from build123d import *

# Parameters (mm, degrees)
F1_DEPTH = 50.8
F3_DEPTH = 76.2
F4_R     = 38.1
F5_DEPTH = 12.7
F6_R     = 9.525
F7_DEPTH = 25.401


with BuildPart() as f1:
    # F0 (on Front) → F1 (new body, symmetric)
    with BuildSketch(Plane.XZ):
        with BuildLine():
            ThreePointArc((-92.075, -61.1803239805), (-60.325, -61.1803239805), (-44.45, -88.6766305507))
            Line((-44.45, -88.6766305507), (44.45, -88.6766305507))
            ThreePointArc((44.45, -88.6766305507), (60.325, -61.1803239805), (92.075, -61.1803239805))
            Line((92.075, -61.1803239805), (159.3117036526, 55.2770628791))
            ThreePointArc((159.3117036526, 55.2770628791), (147.6903970824, 66.8983694493), (143.4367036526, 82.7733694493))
            Line((143.4367036526, 82.7733694493), (-143.4367036526, 82.7733694493))
            ThreePointArc((-143.4367036526, 82.7733694493), (-147.6903970824, 66.8983694493), (-159.3117036526, 55.2770628791))
            Line((-159.3117036526, 55.2770628791), (-92.075, -61.1803239805))
        make_face()
        with BuildLine():
            Line((-168.8367036526, 71.7748468212), (-159.3117036526, 55.2770628791))
            ThreePointArc((-159.3117036526, 55.2770628791), (-147.6903970824, 66.8983694493), (-143.4367036526, 82.7733694493))
            Line((-143.4367036526, 82.7733694493), (-162.4867036526, 82.7733694493))
            ThreePointArc((-162.4867036526, 82.7733694493), (-164.1881810245, 76.4233694493), (-168.8367036526, 71.7748468212))
        make_face()
        with BuildLine():
            ThreePointArc((-143.4367036526, 82.7733694493), (-202.6830102227, 98.6483694493), (-159.3117036526, 55.2770628791))
            Line((-159.3117036526, 55.2770628791), (-168.8367036526, 71.7748468212))
            ThreePointArc((-168.8367036526, 71.7748468212), (-186.1852262806, 89.1233694493), (-162.4867036526, 82.7733694493))
            Line((-162.4867036526, 82.7733694493), (-143.4367036526, 82.7733694493))
        make_face()
        with BuildLine():
            Line((168.8367036526, 71.7748468212), (159.3117036526, 55.2770628791))
            ThreePointArc((159.3117036526, 55.2770628791), (191.0617036526, 55.2770628791), (206.9367036526, 82.7733694493))
            ThreePointArc((206.9367036526, 82.7733694493), (175.1867036526, 114.5233694493), (143.4367036526, 82.7733694493))
            Line((143.4367036526, 82.7733694493), (162.4867036526, 82.7733694493))
            ThreePointArc((162.4867036526, 82.7733694493), (175.1867036526, 95.4733694493), (187.8867036526, 82.7733694493))
            ThreePointArc((187.8867036526, 82.7733694493), (181.5367036526, 71.7748468212), (168.8367036526, 71.7748468212))
        make_face()
        with BuildLine():
            ThreePointArc((143.4367036526, 82.7733694493), (147.6903970824, 66.8983694493), (159.3117036526, 55.2770628791))
            Line((159.3117036526, 55.2770628791), (168.8367036526, 71.7748468212))
            ThreePointArc((168.8367036526, 71.7748468212), (164.1881810245, 76.4233694493), (162.4867036526, 82.7733694493))
            Line((162.4867036526, 82.7733694493), (143.4367036526, 82.7733694493))
        make_face()
        with BuildLine():
            Line((63.5, -88.6766305507), (44.45, -88.6766305507))
            ThreePointArc((44.45, -88.6766305507), (76.2, -120.4266305507), (107.95, -88.6766305507))
            ThreePointArc((107.95, -88.6766305507), (103.6963065702, -72.8016305507), (92.075, -61.1803239805))
            Line((92.075, -61.1803239805), (82.55, -77.6781079226))
            ThreePointArc((82.55, -77.6781079226), (87.1985226281, -82.3266305507), (88.9, -88.6766305507))
            ThreePointArc((88.9, -88.6766305507), (76.2, -101.3766305507), (63.5, -88.6766305507))
        make_face()
        with BuildLine():
            ThreePointArc((92.075, -61.1803239805), (60.325, -61.1803239805), (44.45, -88.6766305507))
            Line((44.45, -88.6766305507), (63.5, -88.6766305507))
            ThreePointArc((63.5, -88.6766305507), (69.85, -77.6781079226), (82.55, -77.6781079226))
            Line((82.55, -77.6781079226), (92.075, -61.1803239805))
        make_face()
        with BuildLine():
            Line((-44.45, -88.6766305507), (-63.5, -88.6766305507))
            ThreePointArc((-63.5, -88.6766305507), (-82.55, -99.6751531788), (-82.55, -77.6781079226))
            Line((-82.55, -77.6781079226), (-92.075, -61.1803239805))
            ThreePointArc((-92.075, -61.1803239805), (-92.075, -116.1729371209), (-44.45, -88.6766305507))
        make_face()
        with BuildLine():
            ThreePointArc((-82.55, -77.6781079226), (-69.85, -77.6781079226), (-63.5, -88.6766305507))
            Line((-63.5, -88.6766305507), (-44.45, -88.6766305507))
            ThreePointArc((-44.45, -88.6766305507), (-60.325, -61.1803239805), (-92.075, -61.1803239805))
            Line((-92.075, -61.1803239805), (-82.55, -77.6781079226))
        make_face()
    extrude(amount=F1_DEPTH, both=True)

    # F2 (on face) → F3 (cut)
    with BuildSketch(Plane.XZ.offset(50.8)):
        Polygon((50.5367805345, -44.2266305507), (123.8602647216, 82.7733694493), (-123.8602647216, 82.7733694493), (-50.5367805345, -44.2266305507), align=None)
    extrude(amount=-F3_DEPTH, mode=Mode.SUBTRACT)

    # F4 (on Front) → F5 (cut, symmetric)
    with BuildSketch(Plane.XZ):
        with Locations((-175.0013381243, 83.766028285)):
            Circle(F4_R)
    extrude(amount=F5_DEPTH, both=True, mode=Mode.SUBTRACT)

    # F6 (on face) → F7 (cut, through all)
    with BuildSketch(Plane.XZ.offset(-25.4)):
        with Locations((-38.1, -6.1266305507)):
            Circle(F6_R)
        with Locations((38.1, -6.1266305507)):
            Circle(F6_R)
    extrude(amount=-F7_DEPTH, mode=Mode.SUBTRACT)


solid = f1.part
For this review, take the finished solid that the model builds, in its own axes (mm). A direction names the side the tool comes from. Give positions to 0.01 mm unless a question says otherwise; leave off trailing zeros. Order: outer loops, then holes, each group sorted by start corner. A loop starts at its lowest first (then second) coordinate and runs counter-clockwise, first axis right, second up. Notation, with made-up numbers: (-7, 21.25) -> (48, 21.25) arc R27 ccw to (48, 45.25) -> close; hole circle Ø10 at (37, -22). An arc over 180 degrees is marked (long way). Write item = value, one per line.
1) We need section A-A, the plane y = -38. Give the boundary of the cut face in (x, z) (3 decimals), and give its area (3 significant figures).
Findings:
outline = (-159.312, 55.277) -> (-92.075, -61.18) arc R31.75 ccw (long way) to (-44.45, -88.677) -> (44.45, -88.677) arc R31.75 ccw (long way) to (92.075, -61.18) -> (159.312, 55.277) arc R31.75 ccw (long way) to (143.437, 82.773) -> (123.86, 82.773) -> (50.537, -44.227) -> (-50.537, -44.227) -> (-123.86, 82.773) -> (-143.437, 82.773) arc R31.75 ccw (long way) to start; hole circle Ø25.4 at (-175.187, 82.773); hole circle Ø25.4 at (-76.2, -88.677); hole circle Ø25.4 at (76.2, -88.677); hole circle Ø25.4 at (175.187, 82.773)
area = 28,400 mm^2
2) We need section D-D, the plane y = 42. Give the boundary of the cut face in (x, z) (3 decimals), and give its area (3 significant figures).
Findings:
outline = (-159.312, 55.277) -> (-92.075, -61.18) arc R31.75 ccw (long way) to (-44.45, -88.677) -> (44.45, -88.677) arc R31.75 ccw (long way) to (92.075, -61.18) -> (159.312, 55.277) arc R31.75 ccw (long way) to (143.437, 82.773) -> (-143.437, 82.773) arc R31.75 ccw (long way) to start; hole circle Ø25.4 at (-175.187, 82.773); hole circle Ø25.4 at (-76.2, -88.677); hole circle Ø19.05 at (-38.1, -6.127); hole circle Ø19.05 at (38.1, -6.127); hole circle Ø25.4 at (76.2, -88.677); hole circle Ø25.4 at (175.187, 82.773)
area = 50,000 mm^2
3) Insertion check: pin 1 (22 mm diameter, centred on x = 38.1, z = -6.13, fed in from -Y); pin 2 (6 mm diameter, centred on y = 18.5, z = 6.5, fed in from +X); pin 3 (5 mm diameter, centred on x = -153, y = 26.5, fed in from -Z); pin 4 (25 mm diameter, centred on x = -38.1, z = -6.13, fed in from +Y). Each pin has a flat end and moves straight along its axis. Give the tip position at first contact, or say it passes through.
Findings:
pin_1 = 25.4
pin_2 = 132.88
pin_3 = 40.01
pin_4 = 50.8
4) For faces 1 (the face through (-164.6, 12.7, 90.1)), 2 (the face through (2, 33, 82.773)), 3 (the face through (-87.71, -13.23, 20.16)), list the 3-axis set-ups (+Z, -Z, +X, -X, +Y, -Y) from which the entire face can be reached by the end or side of a thin tool; tool diameter is ignored.
Findings:
face_1 = +Z, -X
face_2 = +Z, +Y, -Y
face_3 = +Z, -Y
5) To check wall thickness, follow L1, parallel to Z at x = -38, y = 44; L2, parallel to Z at x = -76.2, y = 26; L3, parallel to X at y = 8, z = 64. State the ranges of each line that lie inside material, in increasing order. Write a range as from..to.
Findings:
L1 = -88.68..-15.65, 3.4..82.77
L2 = -120.43..-101.38, -75.98..82.77
L3 = -142.43..-113.02, 113.02..200.79
6) We need section B-B, the plane x = -38.1. Give the boundary of the cut face in (y, z), and give its area (3 significant figures).
Findings:
outline = (-50.8, -88.68) -> (50.8, -88.68) -> (50.8, -15.65) -> (25.4, -15.65) -> (25.4, -44.23) -> (-50.8, -44.23) -> close; (25.4, 3.4) -> (50.8, 3.4) -> (50.8, 82.77) -> (25.4, 82.77) -> close
area = 7,260 mm^2
7) We need section C-C, the plane z = 17. Give the boundary of the cut face in (x, y), and give its area (3 significant figures).
Findings:
outline = (-137.21, -50.8) -> (-85.89, -50.8) -> (-85.89, 25.4) -> (85.89, 25.4) -> (85.89, -50.8) -> (137.21, -50.8) -> (137.21, 50.8) -> (-137.21, 50.8) -> close
area = 14,800 mm^2
8) Draft analysis for pull direction Z (two halves, no side actions). For faces 4 (the face through (125.22, -0.71, -3.77)), 5 (the face through (-1, -50.8, -46)), 6 (the face through (203.246, -0.711, 97.63)), state which applies: pulls with the +Z half, pulls with the -Z half, needs draft (parallel to the pull), parting line crosses it, or undercut.
Findings:
face_4 = undercut
face_5 = needs draft
face_6 = parting line crosses it
